Part print with two shaded views. Sizes in mm from the minimum x, y, z corner. Give positions to 0.01 mm unless a question says otherwise; leave off trailing zeros. Order: outer loops, then holes, each group sorted by start corner. A loop starts at its lowest first (then second) coordinate and runs counter-clockwise, first axis right, second up. Notation, with made-up numbers: M -10,14 L 0,14 A16 cw 0,34 Z; hole C -22,-36 d2. An arc over 180 degrees is marked long. Return JSON: item names as keys, results as strings. Group by question number.
1. Slice it at D-D on z = 16.75. List the corners of the cut face in (x, y), then the cut area to 3 significant figures.
2. Pin check, flat tips, straight feed: pin 1 (1 mm diameter, centred on x = 2, z = 11, fed in from +Y); pin 2 (1.5 mm diameter, centred on x = 5, z = 12.5, fed in from -Y); pin 3 (4 mm diameter, centred on x = 1.5, z = 2.5, fed in from -Y). Stop position of each tip, or through.
3. Slice it at A-A on y = 9.5. List the corners of the cut face in (x, z), then the cut area to 3 significant figures.
4. Wall check: probe 1 along Z at (x, y) = (6, 14); probe 2 along Y at (x, z) = (4, 10.25); probe 3 along Z at (x, y) = (2.25, 10). Give the ranges that are in metal, low to high. Write a range as [from, to].
5. Slice it at C-C on x = 1.75. List the corners of the cut face in (y, z), then the cut area to 3 significant figures.
6. Two-plate mould, pull along Y, no slides. Class the marked faces 1, 2, 3 and 4: released by +Y, released by -Y, zero draft, split by the parting line, or undercut.
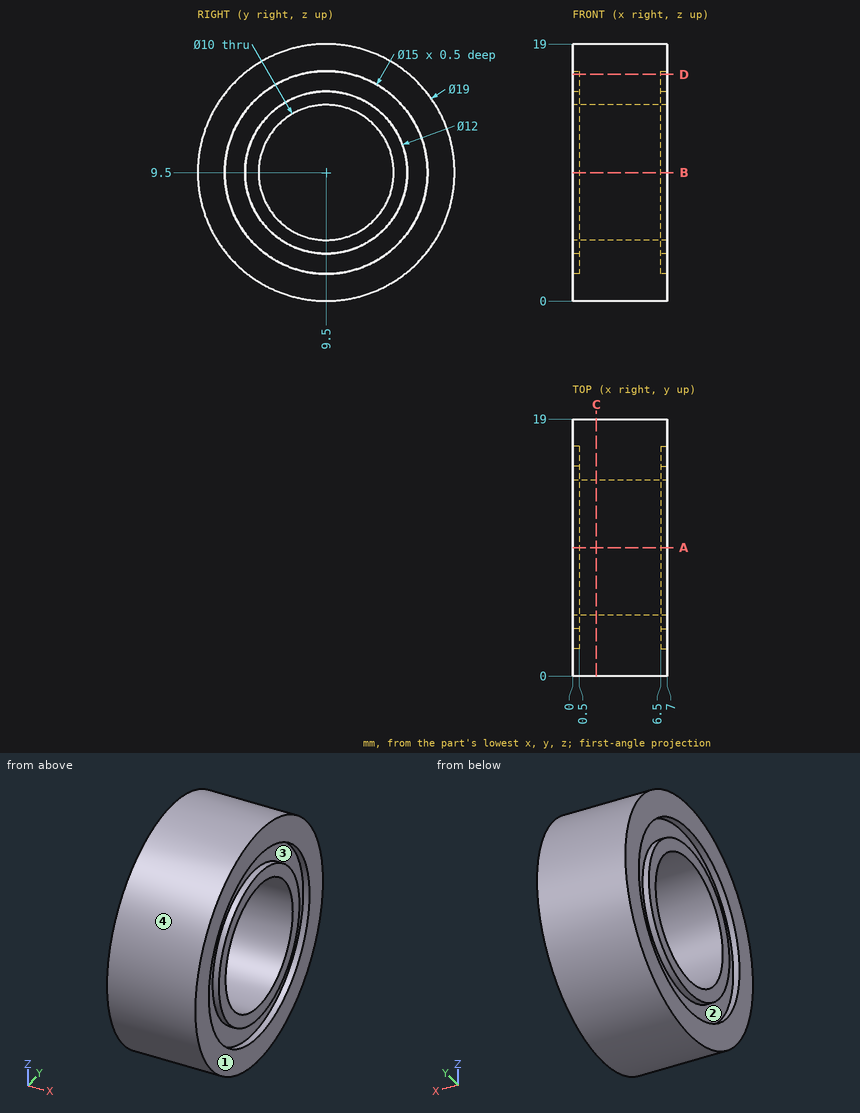
Result:
{
 "1": {"outline": "M 0,3.36 L 7,3.36 L 7,7.58 L 6.5,7.58 L 6.5,11.42 L 7,11.42 L 7,15.64 L 0,15.64 L 0,11.42 L 0.5,11.42 L 0.5,7.58 L 0,7.58 Z", "area": "82.1 mm2"},
 "2": {"pin 1": "stops at y = 18.95", "pin 2": "stops at y = 0.27", "pin 3": "stops at y = 1.42"},
 "3": {"outline": "M 0,0 L 7,0 L 7,2 L 6.5,2 L 6.5,3.5 L 7,3.5 L 7,4.5 L 0,4.5 L 0,3.5 L 0.5,3.5 L 0.5,2 L 0,2 Z; M 0,14.5 L 7,14.5 L 7,15.5 L 6.5,15.5 L 6.5,17 L 7,17 L 7,19 L 0,19 L 0,17 L 0.5,17 L 0.5,15.5 L 0,15.5 Z", "area": "60.0 mm2"},
 "4": {"probe 1": "z = [1.13, 7.32], [11.68, 17.87]", "probe 2": "y = [0.03, 4.56], [14.44, 18.97]", "probe 3": "z = [0.01, 4.53], [14.47, 18.99]"},
 "5": {"outline": "C 9.5,9.5 d19; hole C 9.5,9.5 d10", "area": "205 mm2"},
 "6": {"face 1": "zero draft", "face 2": "undercut", "face 3": "undercut", "face 4": "split by the parting line"}
}
